```python
from build123d import *

# Parameters (mm, degrees)
ESQUISSE1_R      = 12
ESQUISSE1_R_2    = 2.5
ESQUISSE1_R_3    = 1.5
EXTRUSION1_DEPTH = 2
CHANFREIN1_SIZE  = 0.5


with BuildPart() as part:
    # Esquisse1 → Extrusion1 (new body)
    with BuildSketch(Plane(origin=(0, 0, 0), x_dir=(1, 0, 0), z_dir=(0, 1, 0))):
        with BuildLine():
            Line((-11.9132867, 51.44), (-17.86993005, 2.16))
            ThreePointArc((-17.86993005, 2.16), (0, -18), (17.86993005, 2.16))
            Line((17.86993005, 2.16), (11.9132867, 51.44))
            ThreePointArc((11.9132867, 51.44), (0, 62), (-11.9132867, 51.44))
        make_face()
        Circle(ESQUISSE1_R, mode=Mode.SUBTRACT)
        with Locations((0, 50)):
            Circle(ESQUISSE1_R_2, mode=Mode.SUBTRACT)
        with Locations((-12.557368355, -7.25)):
            Circle(ESQUISSE1_R_3, mode=Mode.SUBTRACT)
        with Locations((12.557368355, -7.25)):
            Circle(ESQUISSE1_R_3, mode=Mode.SUBTRACT)
        with Locations((0, 14.5)):
            Circle(ESQUISSE1_R_3, mode=Mode.SUBTRACT)
    extrude(amount=EXTRUSION1_DEPTH)

    # Chanfrein1
    chanfrein1_edges = [part.edges().sort_by_distance(p)[0] for p in [
        (-12, 0, 0),
        (-12, 2, 0),
        (-2.5, 0, -50),
        (-2.5, 2, -50),
    ]]
    chamfer(chanfrein1_edges, length=CHANFREIN1_SIZE)


solid = part.part
```
Check sheet for the modelled part. Datum: model origin and axes. Units: mm. Round coordinates to 2 decimals unless told otherwise and drop trailing zeros. Loops run counter-clockwise (first coordinate to the right, second up) from the corner with the lowest first, then second, coordinate; pieces in that order, holes last. Notation, with made-up numbers: (51, -11) - (94, -11) arc R24 ccw to (94, 4) - close; hole circle Ø5 at (11.25, -22.75). An arc over 180 degrees is marked (long way). Write item = value, one per line. Start each with the question number.
Q1. Release check for a two-part mould opening along Z. For faces 1 (the face through (0, 1, -62)), 2 (the face through (0, 0, -23)), 3 (the face through (-11.99, 0.99, -0.53)) record: pulls with the +Z half, pulls with the -Z half, needs draft (parallel to the pull), parting line crosses it, or undercut.
Q2. Section check B-B (z = 0). Record the boundary of the cut face in (x, y), plus the area to 3 significant figures.
Q3. Section check D-D (x = -15). Record the boundary of the cut face in (y, z), plus the area to 3 significant figures.
Q4. Section check C-C (z = -50). Record the boundary of the cut face in (x, y).
Q5. Thickness scan on L1, parallel to Z at x = 0, y = 0.75; L2, parallel to X at y = 0.85, z = 0; L3, parallel to X at y = 0.65, z = 7.25. Record the ranges inside material, lowest first.
Q6. Depth check by flat-ended pin: P1, Ø6, axis at x = -12.5, z = -53, coming from the -Y side; P2, Ø1, axis at x = 5, y = 1.5, coming from the -Z side; P3, Ø2.5, axis at x = 0, z = -14.5, coming from the +Y side. Enter the tip coordinate at first touch or a pass-through.
Q7. Section check A-A (x = 0). Record the boundary of the cut face in (y, z), plus the area to 3 significant figures.
Derived:
q1.face_1 = pulls with the -Z half
q1.face_2 = needs draft
q1.face_3 = undercut
q2.outline = (-18, 0) - (-12.5, 0) - (-12, 0.5) - (-12, 1.5) - (-12.5, 2) - (-18, 2) - close; (12, 0.5) - (12.5, 0) - (18, 0) - (18, 2) - (12.5, 2) - (12, 1.5) - close
q2.area = 23.5 mm^2
q3.outline = (0, -25.9) - (2, -25.9) - (2, 9.95) - (0, 9.95) - close
q3.area = 71.7 mm^2
q4.outline = (-12.09, 0) - (-3, 0) - (-2.5, 0.5) - (-2.5, 1.5) - (-3, 2) - (-12.09, 2) - close; (2.5, 0.5) - (3, 0) - (12.09, 0) - (12.09, 2) - (3, 2) - (2.5, 1.5) - close
q5.L1 = -62 to -52.5, -47.5 to -16, -13 to -12, 12 to 18
q5.L2 = -18 to -12, 12 to 18
q5.L3 = -16.48 to -14.06, -11.06 to -9.56, 9.56 to 11.06, 14.06 to 16.48
q6.P1 = 0
q6.P2 = -61.12
q6.P3 = through
q7.outline = (0, -62) - (2, -62) - (2, -53) - (1.5, -52.5) - (0.5, -52.5) - (0, -53) - close; (0, -47) - (0.5, -47.5) - (1.5, -47.5) - (2, -47) - (2, -16) - (0, -16) - close; (0, -13) - (2, -13) - (2, -12.5) - (1.5, -12) - (0.5, -12) - (0, -12.5) - close; (0, 12.5) - (0.5, 12) - (1.5, 12) - (2, 12.5) - (2, 18) - (0, 18) - close
q7.area = 95.0 mm^2
